The listing builds one solid part. Answer for the finished solid, in the listing's coordinates (mm). Face numbers are marked on the shaded views. Round coordinates to 2 decimals unless told otherwise and drop trailing zeros. Write each loop counter-clockwise with the first axis right and the second up, starting at its lowest first coordinate (ties: lowest second). Pieces come first, ordered by that corner, then holes. Notation, with made-up numbers: (-5, 77) - (47, 77) arc R13 cw to (47, 95) - close; hole circle Ø10 at (28.5, 87.5). An arc over 180 degrees is marked (long way). Use a Markdown table: item, result. Add a question column.
1) Determine the mould class of the marked faces 1, 2, 3 and 4 for opening direction X: +X half, -X half, draft (parallel to the pull), parting line (faces both ways), or undercut.
2) Find the intervals of material crossed by probe 1 along X at (y, z) = (23, 0); probe 2 along X at (y, z) = (4, 2); probe 3 along Z at (x, y) = (1, 6), in increasing order. Write a range as from..to.
3) Each of these flat-tipped pins is pushed along its axis until it touches: P1, Ø3, axis at y = 4.5, z = -21, coming from the +X side; P2, Ø1.5, axis at x = 22, z = -9, coming from the -Y side; P3, Ø5, axis at y = 29, z = -6.5, coming from the -X side; P4, Ø3, axis at y = 25.5, z = 4, coming from the -X side. Where does it stop, or does it pass through?
4) A cutting plane is placed at C-C (z = 12). Give the vertices of the cut face in (x, y), then the cut area to 3 significant figures.
5) A cutting plane is placed at B-B (y = 9). Give the vertices of the cut face in (x, z), then the cut area to 3 significant figures.
6) A cutting plane is placed at A-A (x = 0). Give the vertices of the cut face in (y, z), then the cut area to 3 significant figures.
7) A cutting plane is placed at D-D (z = -16.5). Give the vertices of the cut face in (x, y), then the cut area to 3 significant figures.
```python
from build123d import *

# Parameters (mm, degrees)
BOSS_EXTRUDE1_DEPTH = 35
SKETCH8_R           = 15
CUT_EXTRUDE1_DEPTH  = 58.662812973


with BuildPart() as part:
    # Sketch1 → Boss-Extrude1 (new body)
    with BuildSketch(Plane(origin=(0, 0, 0), x_dir=(1, 0, 0), z_dir=(0, 1, 0))):
        Polygon((-17.320508076, -30), (17.320508076, -30), (34.641016151, 0), (-34.641016151, 0), align=None)
        Polygon((-34.641016151, 0), (34.641016151, 0), (17.320508076, 30), (-17.320508076, 30), align=None)
    extrude(amount=BOSS_EXTRUDE1_DEPTH)

    # Sketch6 → Cut-Revolve2 (revolve, cut)
    with BuildSketch(Plane.XY):
        Polygon((30.641016151, 35), (34.641016151, 31), (34.641016151, 35), align=None)
    revolve(axis=Axis((0, 42.436882795, 0), (0, -1, 0)), mode=Mode.SUBTRACT)

    # Sketch8 → Cut-Extrude1 (cut, through all)
    with BuildSketch(Plane(origin=(0, 0, 0), x_dir=(-1, 0, 0), z_dir=(0, -1, 0))):
        with Locations(Location((0, 0, 0), (0, 0, 90))):
            Circle(SKETCH8_R)
    extrude(amount=-CUT_EXTRUDE1_DEPTH, mode=Mode.SUBTRACT)


solid = part.part
```
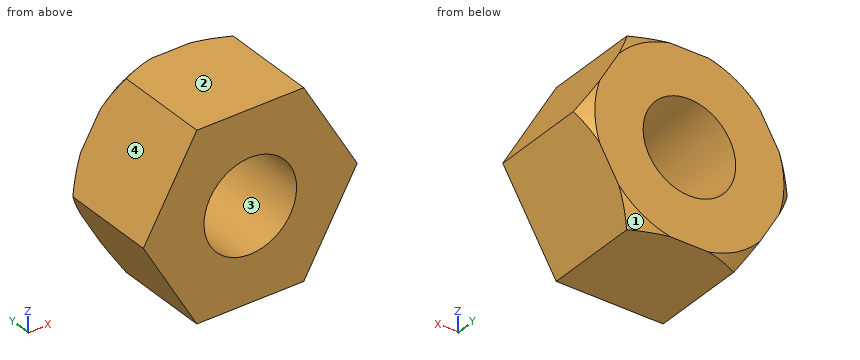
Entries:
| question | item | result |
|---|---|---|
| 1 | face 1 | +X half |
| 1 | face 2 | draft |
| 1 | face 3 | undercut |
| 1 | face 4 | -X half |
| 2 | probe 1 | x = -34.64..-15, 15..34.64 |
| 2 | probe 2 | x = -33.49..-14.87, 14.87..33.49 |
| 2 | probe 3 | z = -30..-14.97, 14.97..30 |
| 3 | P1 | stops at x = 23.38 |
| 3 | P2 | stops at y = 0 |
| 3 | P3 | stops at x = -32.33 |
| 3 | P4 | stops at x = -33.2 |
| 4 | outline | (-27.71, 0) - (-9, 0) - (-9, 35) - (-27.71, 35) - close; (9, 0) - (27.71, 0) - (27.71, 35) - (9, 35) - close |
| 4 | area | 1,310 mm² |
| 5 | outline | (-34.64, 0) - (-17.32, -30) - (17.32, -30) - (34.64, 0) - (17.32, 30) - (-17.32, 30) - close; hole circle Ø30 at (0, 0) |
| 5 | area | 2,410 mm² |
| 6 | outline | (0, -30) - (35, -30) - (35, -15) - (0, -15) - close; (0, 15) - (35, 15) - (35, 30) - (0, 30) - close |
| 6 | area | 1,050 mm² |
| 7 | outline | (-25.11, 0) - (25.11, 0) - (25.11, 35) - (-25.11, 35) - close |
| 7 | area | 1,760 mm² |
